from build123d import *

# Parameters (mm, degrees)
BOSS_EXTRUDE1_DEPTH                 = 8.89
F_2_56_TAPPED_HOLE1_D               = 1.778
F_2_56_TAPPED_HOLE1_DEPTH           = 2.54
F_2_56_TAPPED_HOLE1_TIP             = 0.53416509
F_2_56_TAPPED_HOLE1_ON_FACE_2_D     = 1.778
F_2_56_TAPPED_HOLE1_ON_FACE_2_DEPTH = 2.54
F_2_56_TAPPED_HOLE1_ON_FACE_2_TIP   = 0.53416509


with BuildPart() as part:
    # Sketch1 → Boss-Extrude1 (new body)
    with BuildSketch(Plane(origin=(0, 0, 0), x_dir=(1, 0, 0), z_dir=(0, 1, 0))):
        with BuildLine():
            Line((6.731, 3.81), (8.89, 3.81))
            Line((8.89, 3.81), (8.89, 0))
            Line((8.89, 0), (0, 0))
            Line((0, 0), (0, 3.81))
            Line((0, 3.81), (5.969, 3.81))
            ThreePointArc((5.969, 3.81), (6.35, 3.429), (6.731, 3.81))
        make_face()
    extrude(amount=BOSS_EXTRUDE1_DEPTH)

    # #2-56 Tapped Hole1
    with Locations(Plane(origin=(8.89, 2.54, -1.905), x_dir=(0, 0, 1), z_dir=(1, 0, 0))):
        with Locations((0, 0), (0, -3.81)):
            Hole(F_2_56_TAPPED_HOLE1_D / 2, depth=F_2_56_TAPPED_HOLE1_DEPTH)
            with Locations((0, 0, -(F_2_56_TAPPED_HOLE1_DEPTH + F_2_56_TAPPED_HOLE1_TIP / 2))):  # 118° drill point
                Cone(0, F_2_56_TAPPED_HOLE1_D / 2, F_2_56_TAPPED_HOLE1_TIP, mode=Mode.SUBTRACT)

    # #2-56 Tapped Hole1 on face 2
    with Locations(Plane(origin=(2.032, 2.54, -3.81), x_dir=(-1, 0, 0), z_dir=(0, 0, -1))):
        with Locations((0, 0), (0, 3.81)):
            Hole(F_2_56_TAPPED_HOLE1_ON_FACE_2_D / 2, depth=F_2_56_TAPPED_HOLE1_ON_FACE_2_DEPTH)
            with Locations((0, 0, -(F_2_56_TAPPED_HOLE1_ON_FACE_2_DEPTH + F_2_56_TAPPED_HOLE1_ON_FACE_2_TIP / 2))):  # 118° drill point
                Cone(0, F_2_56_TAPPED_HOLE1_ON_FACE_2_D / 2, F_2_56_TAPPED_HOLE1_ON_FACE_2_TIP, mode=Mode.SUBTRACT)


solid = part.part
Check sheet for the modelled part. Datum: model origin and axes. Units: mm. A direction names the side the tool comes from. Round coordinates to 2 decimals unless told otherwise and drop trailing zeros. Loops run counter-clockwise (first coordinate to the right, second up) from the corner with the lowest first, then second, coordinate; pieces in that order, holes last.
1. Sectioned sample at A-A on x = 7.5. Record the boundary of the cut face in (y, z) (3 decimals), and give its area (3 significant figures).
2. Mould release check, pull along X, two halves, no side actions. Record for faces 4 (the flat face through (3, 4, -3.81)), 5 (the conical face through (5.91, 2.63, -2.03)), 6 (the cylindrical face through (2.44, 1.75, -2.52)), 7 (the flat face through (0, 4, -2)): released by +X, released by -X, zero draft, split by the parting line, or undercut.
3. Set-up check for faces 1 (the cylindrical face through (1.92, 7.23, -2.52)), 2 (the flat face through (8.89, 4, -2)), 3 (the cylindrical face through (7.6, 1.66, -1.79)): record each of +Z, -Z, +X, -X, +Y, -Y from which the full face is reachable in a straight line by a thin tool's end or side.
4. Scan lines: probe 1 along Z at (x, y) = (7.1, 6.35); probe 2 along Y at (x, z) = (1.5, -2.1); probe 3 along Y at (x, z) = (1.25, -1.5). Record each from-to range of solid material in increasing order.
5. Sectioned sample at B-B on x = 6.5. Record the boundary of the cut face in (y, z) (3 decimals).
Recorded:
1. outline: (0, -3.81) - (8.89, -3.81) - (8.89, 0) - (0, 0) - close; hole circle Ø1.778 at (2.54, -1.905); hole circle Ø1.778 at (6.35, -1.905)
1. area: 28.9 mm2
2. face 4: zero draft
2. face 5: released by +X
2. face 6: undercut
2. face 7: released by -X
3. face 1: -Z
3. face 2: +Z, -Z, +X, +Y, -Y
3. face 3: +X
4. probe 1: z = -3.81 to -2.79, -1.02 to 0
4. probe 2: y = 0 to 1.83, 3.25 to 5.64, 7.06 to 8.89
4. probe 3: y = 0 to 2.12, 2.96 to 5.93, 6.77 to 8.89
5. outline: (0, -3.46) - (8.89, -3.46) - (8.89, 0) - (0, 0) - close; hole circle Ø1.778 at (2.54, -1.905); hole circle Ø1.778 at (6.35, -1.905)
